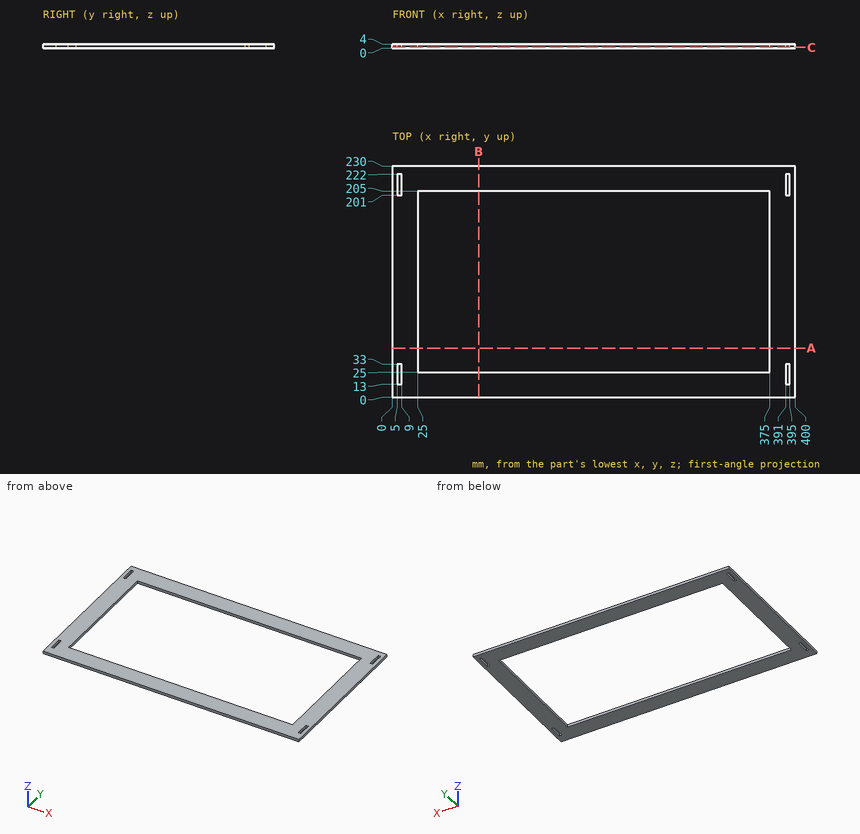
The drawing under review shows one solid part. Ordinate dimensions are in mm from its lowest x, y, z. Give positions to 0.01 mm unless a question says otherwise; leave off trailing zeros. Write each loop counter-clockwise with the first axis right and the second up, starting at its lowest first coordinate (ties: lowest second). Pieces come first, ordered by that corner, then holes. Notation, with made-up numbers: (-27, -16) -> (17, -16) arc R32 cw to (17, 15) -> close; hole circle Ø10 at (3.25, 48). An arc over 180 degrees is marked (long way). Use CSV: the item, a comma, the result in double quotes.
Q1. Take a section at B-B, the plane x = 85.5. Write out the cut boundary in (y, z), then the cut area to 3 significant figures.
Conclusion:
outline,"(0, 0) -> (25, 0) -> (25, 4) -> (0, 4) -> close; (205, 0) -> (230, 0) -> (230, 4) -> (205, 4) -> close"
area,"200 mm2"
Q2. Take a section at A-A, the plane y = 49. Write out the cut boundary in (x, z).
Conclusion:
outline,"(0, 0) -> (25, 0) -> (25, 4) -> (0, 4) -> close; (375, 0) -> (400, 0) -> (400, 4) -> (375, 4) -> close"
Q3. For P1, Ø2, axis at x = 392.5, z = 2.5, coming from the -Y side, flat-tipped, find the tip position at first contact; note if it passes through.
Conclusion:
P1,"y = 0"
Q4. Take a section at C-C, the plane z = 0.7. Write out the cut boundary in (x, y).
Conclusion:
outline,"(0, 0) -> (400, 0) -> (400, 230) -> (0, 230) -> close; hole (5, 13) -> (9, 13) -> (9, 33) -> (5, 33) -> close; hole (5, 201) -> (9, 201) -> (9, 222) -> (5, 222) -> close; hole (25, 25) -> (375, 25) -> (375, 205) -> (25, 205) -> close; hole (391, 13) -> (395, 13) -> (395, 33) -> (391, 33) -> close; hole (391, 201) -> (395, 201) -> (395, 222) -> (391, 222) -> close"
Q5. To check wall thickness, follow probe 1 along X at (y, z) = (24, 3.65); probe 2 along Y at (x, z) = (171.5, 2.4); probe 3 along X at (y, z) = (184, 3.15). State the ranges of each line that lie inside material, in increasing order. Write a range as [from, to].
Conclusion:
probe 1,"[0, 5], [9, 391], [395, 400]"
probe 2,"[0, 25], [205, 230]"
probe 3,"[0, 25], [375, 400]"
